Part model, mm, in its own coordinate system. A direction names the side the tool comes from. Give positions to 0.01 mm unless a question says otherwise; leave off trailing zeros. Order: outer loops, then holes, each group sorted by start corner. A loop starts at its lowest first (then second) coordinate and runs counter-clockwise, first axis right, second up. Notation, with made-up numbers: M 54,80 L 87,80 A27 cw 87,97 Z; hole C 76.25,87 d9. An arc over 180 degrees is marked long. Answer as a JSON object with one key per item and string values.
from build123d import *

# Parameters (mm, degrees)
BOSS_EXTRUDE1_DEPTH              = 50.8
F_9_0_196_DIAMETER_HOLE2_D       = 4.9784
F_9_0_196_DIAMETER_HOLE3_D       = 4.9784
F_1_8_0_125_DIAMETER_HOLE1_D     = 3.175
F_1_8_0_125_DIAMETER_HOLE1_DEPTH = 3.302


with BuildPart() as part:
    # Sketch1 → Boss-Extrude1 (new body)
    with BuildSketch(Plane.XY):
        Polygon((0, 0), (0, 32.004), (23.114, 32.004), (23.114, 28.829), (3.302, 28.829), (3.302, 0), align=None)
    extrude(amount=BOSS_EXTRUDE1_DEPTH)

    # #9 (0.196) Diameter Hole2 (through all)
    with Locations(Plane(origin=(0, 32.004, 0), x_dir=(1, 0, 0), z_dir=(0, 1, 0))):
        with Locations((13.280812395, -26.046570346), (13.280812395, -6.366207965), (13.280812395, -43.514069015)):
            Hole(F_9_0_196_DIAMETER_HOLE2_D / 2)

    # #9 (0.196) Diameter Hole3 (through all)
    with Locations(Plane.ZY):
        with Locations((6.2896856, 18.761683292), (26.205635925, 18.761683292), (43.966936654, 18.761683292)):
            Hole(F_9_0_196_DIAMETER_HOLE3_D / 2)

    # 1/8 (0.125) Diameter Hole1
    with Locations(Plane.ZY):
        with Locations((36.442896127, 16.028307276), (33.392991473, 7.842756721), (25.109056897, 4.694468046), (16.884152733, 7.842756721), (13.794894471, 16.028307276), (16.884152733, 24.292565048), (25.109056897, 27.362146507), (33.392991473, 24.292565048)):
            Hole(F_1_8_0_125_DIAMETER_HOLE1_D / 2, depth=F_1_8_0_125_DIAMETER_HOLE1_DEPTH)


solid = part.part
1. Cut at C-C on x = 15.25. Give the cut face in (y, z).
Worked answers:
{"outline": "M 28.83,0 L 32,0 L 32,4.84 L 28.83,4.84 Z; M 28.83,7.89 L 32,7.89 L 32,24.52 L 28.83,24.52 Z; M 28.83,27.57 L 32,27.57 L 32,41.99 L 28.83,41.99 Z; M 28.83,45.04 L 32,45.04 L 32,50.8 L 28.83,50.8 Z"}
2. Cut at A-A on y = 30. Give the cut face in (x, z), plus the area to 3 significant figures.
Worked answers:
{"outline": "M 0,0 L 23.11,0 L 23.11,50.8 L 0,50.8 Z; hole C 13.28,6.37 d4.98; hole C 13.28,26.05 d4.98; hole C 13.28,43.51 d4.98", "area": "1,120 mm^2"}
3. Which spindle directions (+Z, -Z, +X, -X, +Y, -Y) get a long thin tool onto all of the face, cutting with end or side? Do faces 1 (the cylindrical face through (1.67, 7.91, 34.98)), 2 (the flat face through (18, 28.829, 25)). Say none if no direction does.
Worked answers:
{"face 1": "+X, -X", "face 2": "+Z, -Z, +X, -Y"}
4. Cut at B-B on z = 7. Give the cut face in (x, y), plus the area to 3 significant figures.
Worked answers:
{"outline": "M 0,0 L 3.3,0 L 3.3,16.38 L 0,16.38 Z; M 0,21.15 L 3.3,21.15 L 3.3,28.83 L 10.87,28.83 L 10.87,32 L 0,32 Z; M 15.69,28.83 L 23.11,28.83 L 23.11,32 L 15.69,32 Z", "area": "138 mm^2"}
5. Probe line 1 along Y through (x, z) = (2.5, 16); line 2 along Y through (x, z) = (8, 43.5); line 3 along X through (y, z) = (9.5, 28.5). List the from-to ranges inside material, lowest first.
Worked answers:
{"line 1": "y = 0 to 6.52, 9.16 to 22.97, 25.61 to 32", "line 2": "y = 28.83 to 32", "line 3": "x = 0 to 3.3"}
6. Cut at D-D on y = 4. Give the cut face in (x, z), plus the area to 3 significant figures.
Worked answers:
{"outline": "M 0,0 L 3.3,0 L 3.3,23.68 L 0,23.68 Z; M 0,26.54 L 3.3,26.54 L 3.3,50.8 L 0,50.8 Z", "area": "158 mm^2"}
7. Two-plate mould, pull along Y, no slides. Class faces 3 (the flat face through (2, 0, 25)), 4 (the cylindrical face through (1.674, 23.327, 34.653)), 5 (the flat face through (9, 32.004, 25)), 6 (the flat face through (3, 22, 50.8)): +Y half, -Y half, draft (parallel to the pull), parting line (faces both ways), or undercut.
Worked answers:
{"face 3": "-Y half", "face 4": "undercut", "face 5": "+Y half", "face 6": "draft"}
8. Pin check, flat tips, straight feed: P1, Ø3, axis at y = 18.76, z = 43.97, coming from the +X side (3 decimals); P2, Ø6.5, axis at x = 13.28, z = 26.05, coming from the +Y side; P3, Ø5, axis at y = 4.69, z = 25.11, coming from the +X side; P4, Ø8, axis at x = 14, z = 12.5, coming from the -Y side. Stop position of each tip, or through.
Worked answers:
{"P1": "passes through", "P2": "stops at y = 32", "P3": "stops at x = 3.3", "P4": "stops at y = 28.83"}
